```python
from build123d import *

# Parameters (mm, degrees)
F0_R     = 320.04
F1_DEPTH = 25.4
F2_R     = 50.79999


# Not quite as in the source:
# - a fillet or chamfer is up to 0.001 mm smaller than in the source, because OpenCascade refuses the exact size


with BuildPart() as f1:
    # F0 (on Top) → F1 (new body)
    with BuildSketch(Plane.XY):
        with BuildLine():
            Line((-50.8, 555.969013028), (-50.8, 454.369013028))
            ThreePointArc((-50.8, 454.369013028), (-323.2892203585, 323.2892203585), (-454.369013028, 50.8))
            Line((-454.369013028, 50.8), (-555.969013028, 50.8))
            Line((-555.969013028, 50.8), (-555.969013028, -50.8))
            Line((-555.969013028, -50.8), (-454.369013028, -50.8))
            ThreePointArc((-454.369013028, -50.8), (-323.2892203585, -323.2892203585), (-50.8, -454.369013028))
            Line((-50.8, -454.369013028), (-50.8, -555.969013028))
            Line((-50.8, -555.969013028), (50.8, -555.969013028))
            Line((50.8, -555.969013028), (50.8, -454.369013028))
            ThreePointArc((50.8, -454.369013028), (323.2892203585, -323.2892203585), (454.369013028, -50.8))
            Line((454.369013028, -50.8), (555.969013028, -50.8))
            Line((555.969013028, -50.8), (555.969013028, 50.8))
            Line((555.969013028, 50.8), (454.369013028, 50.8))
            ThreePointArc((454.369013028, 50.8), (323.2892203585, 323.2892203585), (50.8, 454.369013028))
            Line((50.8, 454.369013028), (50.8, 555.969013028))
            Line((50.8, 555.969013028), (-50.8, 555.969013028))
        make_face()
        Circle(F0_R, mode=Mode.SUBTRACT)
    extrude(amount=F1_DEPTH)

    # F2 (radius 50.8 in the source; OpenCascade refuses exactly that, so slightly less here)
    f2_edges = [f1.edges().sort_by_distance(p)[0] for p in [
        (50.8, -555.969013, 12.7),
        (-50.8, -555.969013, 12.7),
        (555.969013, -50.8, 12.7),
        (555.969013, 50.8, 12.7),
        (50.8, 555.969013, 12.7),
        (-50.8, 555.969013, 12.7),
        (-555.969013, 50.8, 12.7),
        (-555.969013, -50.8, 12.7),
        (50.8, -454.369013, 12.7),
        (454.369013, -50.8, 12.7),
        (454.369013, 50.8, 12.7),
        (50.8, 454.369013, 12.7),
        (-50.8, 454.369013, 12.7),
        (-454.369013, 50.8, 12.7),
        (-454.369013, -50.8, 12.7),
        (-50.8, -454.369013, 12.7),
    ]]
    fillet(f2_edges, radius=F2_R)


solid = f1.part
```
Here's how the part is built. I have some questions about the finished solid (model axes, mm). Coordinates: 2 decimals unless noted, no trailing zeros. Order: outer loops, then holes, each group sorted by start corner. A loop starts at its lowest first (then second) coordinate and runs counter-clockwise, first axis right, second up. Notation, with made-up numbers: M -10.5,68 L 40.5,68 A19 ccw 40.5,103 Z; hole C 9.5,36 d8. An arc over 180 degrees is marked long. Answer as a JSON object with one key per item and string values. Group by question number.
(1) Suppose I cut it at D-D, the plane x = 409.5. Please give me the cut outline in (y, z), then the cut area to 3 significant figures.
(2) For pin 1 (2 mm diameter, centred on y = -500, z = 10, fed in from +X); pin 2 (3.5 mm diameter, centred on y = 501.5, z = 11.5, fed in from -X); pin 3 (1 mm diameter, centred on y = -136, z = 14, fed in from -X); pin 4 (2 mm diameter, centred on x = 389.5, y = 77.5, fed in from -Z), each with a flat end and sliding along its axis, tell me the tip position at first contact or that it passes through.
(3) Suppose I cut it at B-B, the plane y = 186.5. Please give me the cut outline in (x, z), then the cut area to 3 significant figures.
(4) If we mould it in two halves opening along Y, with no side actions, what happens to faces 1 (the face through (-209, 250, 25.4)), 2 (the face through (-541.483, -35.524, 12.878)), 3 (the face through (305.26, 96.13, 12.52))? For each: released by +Y, released by -Y, zero draft, split by the parting line, or undercut.
(5) I need wall thicknesses on probe 1 along X at (y, z) = (-210, 8.5); probe 2 along X at (y, z) = (-74, 5.25); probe 3 along Y at (x, z) = (333.5, 12). Which ranges of each line are inside material? Lowest first, please.
(6) Suppose I cut it at C-C, the plane y = 71.5. Please give me the cut outline in (x, z).
Values found:
{
 "1": {"outline": "M -203.33,0 L 203.33,0 L 203.33,25.4 L -203.33,25.4 Z", "area": "10,300 mm^2"},
 "2": {"pin 1": "stops at x = 50.8", "pin 2": "stops at x = -50.8", "pin 3": "stops at x = -436.66", "pin 4": "stops at z = 0"},
 "3": {"outline": "M -417.43,0 L -260.08,0 L -260.08,25.4 L -417.43,25.4 Z; M 260.08,0 L 417.43,0 L 417.43,25.4 L 260.08,25.4 Z", "area": "7,990 mm^2"},
 "4": {"face 1": "zero draft", "face 2": "released by -Y", "face 3": "undercut"},
 "5": {"probe 1": "x = -406.12 to -241.51, 241.51 to 406.12", "probe 2": "x = -455.09 to -311.37, 311.37 to 455.09", "probe 3": "y = -312.75 to 312.75"},
 "6": {"outline": "M -456.81,0 L -311.95,0 L -311.95,25.4 L -456.81,25.4 Z; M 311.95,0 L 456.81,0 L 456.81,25.4 L 311.95,25.4 Z"}
}
